Autodesk Inventor part; units mm, degrees
ref_plane "YZ Plane" through (0, 0, 0) normal (1, 0, 0) x (0, 1, 0)
ref_plane "XZ Plane" through (0, 0, 0) normal (0, 1, 0) x (-1, 0, 0)
ref_plane "XY Plane" through (0, 0, 0) normal (0, 0, 1) x (1, 0, 0)
sketch "Skizze1" plane through (0, 0, 0) normal (0, 0, 1) x (1, 0, 0)
  line L0 (0, 0) -> (50, 0)
  line L1 (50, 0) -> (50, 15)
  line L2 (50, 15) -> (0, 15)
  line L3 (0, 15) -> (0, 0)
  dimension "d0" = 15
  dimension "d1" = 50
extrude "Extrusion1" add sketch "Skizze1" along normal blind 28.5
hole "Bohrung1" at (45, 10, 28.5) direction (0, 0, -1) diameter 3.4 end through all counterbore diameter 6.5 counterbore depth 3
hole "Bohrung2" at (5, 10, 28.5) direction (0, 0, -1) diameter 3.4 end through all counterbore diameter 6.5 counterbore depth 3
chamfer "Fase1" distance 0.5 angle 45 1 edges at (25, 0, 28.5)
sketch "Skizze2" plane through (0, 0, 0) normal (0, 0, -1) x (-1, 0, 0)
  line L0 (0, 15) -> (0, 0)
  line L1 (-50, 15) -> (0, 15)
  line L2 (-50, 0) -> (-50, 15)
  line L3 (-40, 15) -> (-10, 15)
  line L4 (-10, 15) -> (-10, 2)
  line L5 (-10, 2) -> (-40, 2)
  line L6 (-40, 2) -> (-40, 15)
  line L7 (0, 0) -> (-50, 0)
  dimension "d25" = 10
  dimension "d26" = 10
  dimension "d44" = 2
extrude "Extrusion2" cut sketch "Skizze2" against normal blind 25.5 contours L4 L5 L6 L1
hole "Bohrung3" at (25, 8.5, 28.5) direction (0, 0, -1) diameter 5 end through all
chamfer "Fase2" distance 2 angle 45 2 edges at (50, 15, 14.25) (0, 15, 14.25)
sketch "Skizze4" plane through (0, 0, 0) normal (0, 0, -1) x (-1, 0, 0)
  line L0 (-50, 0) -> (-50, 13)
  line L1 (-50, 0) -> (-50, 13)
  line L2 (-50, 13) -> (-48, 15)
  line L3 (-48, 15) -> (-50, 13)
  line L4 (-48, 15) -> (-40, 15)
  line L5 (-48, 15) -> (-40, 15)
  line L6 (-40, 15) -> (-40, 3)
  line L7 (-40, 2) -> (-40, 15)
  line L8 (-40, 2) -> (-10, 2)
  line L9 (-10, 2) -> (-40, 2)
  line L10 (-10, 2) -> (-10, 15)
  line L11 (-10, 15) -> (-10, 2)
  line L12 (-10, 15) -> (-2, 15)
  line L13 (-2, 15) -> (0, 13)
  line L14 (0, 13) -> (-2, 15)
  line L15 (0, 13) -> (0, 0)
  line L16 (0, 0) -> (-50, 0)
  line L17 (0, 0) -> (-50, 0)
extrude "Extrusion4" cut sketch "Skizze4" against normal blind 1.5
properties part number "Peripherie2_Motor2_liegend"
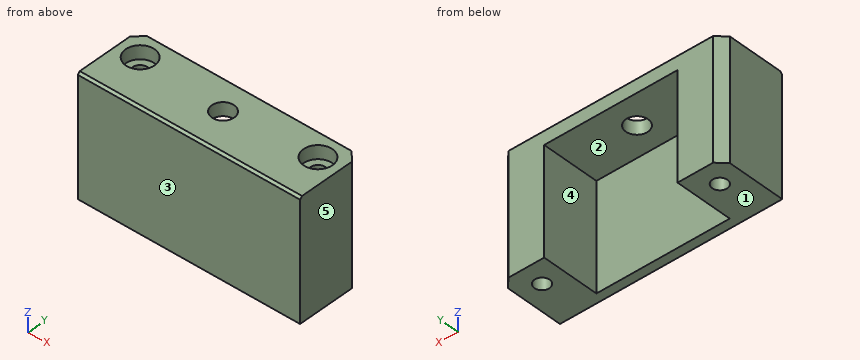
Geometry: final body of the model. Coordinates: model frame, mm. Face numbers are marked on the shaded views. A direction names the side the tool comes from. Round coordinates to 2 decimals unless told otherwise and drop trailing zeros. Loops run counter-clockwise (first coordinate to the right, second up) from the corner with the lowest first, then second, coordinate; pieces in that order, holes last.
Q1. Section B-B on z = 15.5. Return loops of the section in (x, y), plus the area to 3 significant figures.
Q2. Access query for the marked faces 1 and 2. Directions: +Z, -Z, +X, -X, +Y, -Y. A direction counts if a zero-diameter tool reaches every point of the face in a straight line with its end or side. Return the directions, or none.
Q3. Pin query (flat end, axial travel): P1, Ø6.5, axis at x = 23.5, y = 7.5, coming from the -Z side; P2, Ø2, axis at x = 16, z = 9, coming from the +Y side; P3, Ø4, axis at x = 25, y = 8.5, coming from the +Z side; P4, Ø5, axis at x = 45, y = 10, coming from the +Z side. Return the tip coordinate at first contact, or that it passes through.
Q4. Section C-C on y = 10. Return loops of the section in (x, z), plus the area to 3 significant figures.
Q5. Section D-D on z = 26.5. Return loops of the section in (x, y), plus the area to 3 significant figures.
Q6. Section A-A on x = 25. Return loops of the section in (y, z), plus the area to 3 significant figures.
Q7. Pull-direction query (X, two-part tool) for the marked faces 3, 4 and 5; classes: released by +X, released by -X, zero draft, split by the parting line, or undercut.
Q8. Material intervals for L1, parallel to X at y = 10, z = 17.75; L2, parallel to X at y = 5.75, z = 18.5; L3, parallel to Y at x = 45, z = 3.5, sorted ascending.
Evaluation:
1. outline: (0, 0) - (50, 0) - (50, 13) - (48, 15) - (40, 15) - (40, 2) - (10, 2) - (10, 15) - (2, 15) - (0, 13) - close; hole circle Ø3.4 at (5, 10); hole circle Ø3.4 at (45, 10)
1. area: 338 mm2
2. face 1: -Z, +X, -X, +Y, -Y
2. face 2: -Z, +Y
3. P1: stops at z = 25.5
3. P2: stops at y = 2
3. P3: passes through
3. P4: stops at z = 25.5
4. outline: (0, 1.5) - (3.3, 1.5) - (3.3, 25.5) - (1.75, 25.5) - (1.75, 28.5) - (0, 28.5) - close; (6.7, 1.5) - (10, 1.5) - (10, 25.5) - (23, 25.5) - (23, 28.5) - (8.25, 28.5) - (8.25, 25.5) - (6.7, 25.5) - close; (27, 25.5) - (40, 25.5) - (40, 1.5) - (43.3, 1.5) - (43.3, 25.5) - (41.75, 25.5) - (41.75, 28.5) - (27, 28.5) - close; (46.7, 1.5) - (50, 1.5) - (50, 28.5) - (48.25, 28.5) - (48.25, 25.5) - (46.7, 25.5) - close
4. area: 416 mm2
5. outline: (0, 0) - (50, 0) - (50, 13) - (48, 15) - (2, 15) - (0, 13) - close; hole circle Ø6.5 at (5, 10); hole circle Ø5 at (25, 8.5); hole circle Ø6.5 at (45, 10)
5. area: 660 mm2
6. outline: (0, 1.5) - (2, 1.5) - (2, 25.5) - (6, 25.5) - (6, 28.5) - (0.5, 28.5) - (0, 28) - close; (11, 25.5) - (15, 25.5) - (15, 28.5) - (11, 28.5) - close
6. area: 77.9 mm2
7. face 3: zero draft
7. face 4: undercut
7. face 5: released by +X
8. L1: x = 0 to 3.3, 6.7 to 10, 40 to 43.3, 46.7 to 50
8. L2: x = 0 to 10, 40 to 50
8. L3: y = 0 to 8.3, 11.7 to 15
